Input: part model. Units: mm. Frame: model coordinates. A direction names the side the tool comes from. Round coordinates to 2 decimals unless told otherwise and drop trailing zeros. Loops run counter-clockwise (first coordinate to the right, second up) from the corner with the lowest first, then second, coordinate; pieces in that order, holes last. Notation, with made-up numbers: (68, 45.25) -> (88, 45.25) arc R18 cw to (88, 51.25) -> close; hole circle Ø6 at (70, -9). An arc over 180 degrees is marked (long way). Answer in a Markdown table with one row per item. Add a question column.
Q1. Reachability of faces 5 (the face through (2, -2, 2.7)), 6 (the face through (2.86, 0.9, 115.9)) from +Z, -Z, +X, -X, +Y, -Y: full face, straight path, thin tool, end or side. Return the list, or none.
Q2. Ray query, L1, parallel to Z at x = -0.25, y = -0.75; L2, parallel to Z at x = 2.5, y = 1.5; L3, parallel to X at y = -0.5, z = 31. Return the intervals inside material, ascending. Write a range as from..to.
Q3. Section A-A, the plane y = -1.5. Output: boundary loops of the cut face in (x, z), and give its area (3 significant figures).
Q4. Section B-B, the plane z = 58.5. Output: boundary loops of the cut face in (x, y), and give its area (3 significant figures).
Q5. Pin query (flat end, axial travel): pin 1 (2 mm diameter, centred on y = -1.5, z = 148, fed in from +X); pin 2 (1.5 mm diameter, centred on x = 1, z = 37, fed in from -Y); pin 3 (3 mm diameter, centred on x = 0, z = 239.5, fed in from +Y). Return the tip coordinate at first contact, or that it passes through.
Q6. Mould query, pull axis Z, two halves, no side actions, for faces 1 (the face through (0, 0, 0)), 2 (the face through (2, 2, 231.5)), 3 (the face through (-0.54, 2.44, 3.09)), 4 (the face through (0, 2.25, 239)). Classes: pulls with the +Z half, pulls with the -Z half, needs draft (parallel to the pull), parting line crosses it, or undercut.
```python
from build123d import *

# Parameters (mm, degrees)
SKETCH1_R           = 3
BOSS_EXTRUDE1_DEPTH = 245
CUT_EXTRUDE2_DEPTH  = 12
M3_TAPPED_HOLE6_D   = 2.5
SKETCH24_W          = 0.8
SKETCH24_H          = 0.5
M3_TAPPED_HOLE7_D   = 2.5
SKETCH28_W          = 0.5
SKETCH28_H          = 0.8


with BuildPart() as part:
    # Sketch1 → Boss-Extrude1 (new body)
    with BuildSketch(Plane.XY):
        Circle(SKETCH1_R)
    extrude(amount=BOSS_EXTRUDE1_DEPTH)

    # Sketch21 → Cut-Extrude2 (cut)
    with BuildSketch(Plane.XY.offset(245)):
        with BuildLine():
            Line((-1.984313483, 2.25), (1.984313483, 2.25))
            ThreePointArc((1.984313483, 2.25), (0, 3), (-1.984313483, 2.25))
        make_face()
    extrude(amount=-CUT_EXTRUDE2_DEPTH, mode=Mode.SUBTRACT)

    # M3 Tapped Hole6 (through all)
    with Locations(Plane(origin=(0, 2.25, 236), x_dir=(0, 0, 1), z_dir=(0, 1, 0))):
        with Locations((0, 0)):
            Hole(M3_TAPPED_HOLE6_D / 2)

    # Sketch24 → Cut-Revolve1 (revolve, cut)
    with BuildSketch(Plane(origin=(0, 0, 0), x_dir=(0, 0, -1), z_dir=(1, 0, 0))):
        with Locations((-231.9, 2.75)):
            Rectangle(SKETCH24_W, SKETCH24_H)
    revolve(axis=Axis((0, 0, 245), (0, 0, -1)), mode=Mode.SUBTRACT)

    # M3 Tapped Hole7 (through all)
    with Locations(Plane(origin=(0, 3.25, 204), x_dir=(0, 0, 1), z_dir=(0, 1, 0))):
        with Locations((0, 0), (-173, 0)):
            Hole(M3_TAPPED_HOLE7_D / 2)

    # Sketch28 → Cut-Revolve2 (revolve, cut)
    with BuildSketch(Plane(origin=(0, 0, 0), x_dir=(1, 0, 0), z_dir=(0, 1, 0))):
        with Locations((2.75, -3.1)):
            Rectangle(SKETCH28_W, SKETCH28_H)
    revolve(axis=Axis((0, 0, 245), (0, 0, -1)), mode=Mode.SUBTRACT)


solid = part.part
```
Answer block:
| question | item | result |
|---|---|---|
| 1 | face 5 | none |
| 1 | face 6 | +Z, -Z |
| 2 | L1 | 0..29.78, 32.22..202.78, 205.22..234.78, 237.22..245 |
| 2 | L2 | 0..2.7, 3.5..231.5, 232.3..245 |
| 2 | L3 | -2.96..-1.25, 1.25..2.96 |
| 3 | outline | (-2.6, 0) -> (2.6, 0) -> (2.6, 2.7) -> (2, 2.7) -> (2, 3.5) -> (2.6, 3.5) -> (2.6, 231.5) -> (2, 231.5) -> (2, 232.3) -> (2.6, 232.3) -> (2.6, 245) -> (-2.6, 245) -> (-2.6, 232.3) -> (-2, 232.3) -> (-2, 231.5) -> (-2.6, 231.5) -> (-2.6, 3.5) -> (-2, 3.5) -> (-2, 2.7) -> (-2.6, 2.7) -> close; hole circle Ø2.5 at (0, 31); hole circle Ø2.5 at (0, 204); hole circle Ø2.5 at (0, 236) |
| 3 | area | 1,260 mm^2 |
| 4 | outline | circle Ø6 at (0, 0) |
| 4 | area | 28.3 mm^2 |
| 5 | pin 1 | x = 2.96 |
| 5 | pin 2 | y = -2.99 |
| 5 | pin 3 | y = 2.25 |
| 6 | face 1 | pulls with the -Z half |
| 6 | face 2 | undercut |
| 6 | face 3 | undercut |
| 6 | face 4 | needs draft |
